from build123d import *

# Parameters (mm, degrees)
F1_DEPTH = 1.5
F3_DEPTH = 6.5
F4_R     = 0.1
F5_R     = 1
F6_R     = 1


# Not quite as in the source:
# - a feature of the source that left no trace in its solid (it failed there, or was rolled back) is left out


with BuildPart() as f1:
    # F0 (on Top) → F1 (new body)
    with BuildSketch(Plane.XY):
        with BuildLine():
            Line((13.5, -3.5), (13.5, 3))
            Line((13.5, 3), (1.7699947357, 3))
            ThreePointArc((1.7699947357, 3), (1.00332674, 2.4581115268), (1.2583103115, 1.5545594745))
            ThreePointArc((1.2583103115, 1.5545594745), (0.6431264076, -1.8937762339), (-1.9447626006, 0.466795916))
            ThreePointArc((-1.9447626006, 0.466795916), (-2.4990001073, 1.3711303598), (-3.4033345511, 0.8168928531))
            ThreePointArc((-3.4033345511, 0.8168928531), (-2.748556438, -2.1668958229), (0, -3.5))
            Line((0, -3.5), (1.7699947357, -3.5))
            Line((1.7699947357, -3.5), (13.5, -3.5))
        make_face()
    extrude(amount=F1_DEPTH)

    # F2 (on face) → F3 (join, through all)
    with BuildSketch(Plane.XZ.offset(3.5)):
        Polygon((5, 0), (3.5, 0), (3.5, -19.5), (13.5, -19.5), (13.5, -18), (5, -18), align=None)
    extrude(amount=-F3_DEPTH)

    # F4
    f4_edges = [f1.edges().sort_by_distance(p)[0] for p in [
        (5, -0.25, 0),
        (5, -0.25, -18),
    ]]
    fillet(f4_edges, radius=F4_R)

    # F5
    f5_edges = [f1.edges().sort_by_distance(p)[0] for p in [
        (3.5, -0.25, 0),
        (3.5, -0.25, -19.5),
    ]]
    fillet(f5_edges, radius=F5_R)

    # F6
    f6_edges = [f1.edges().sort_by_distance(p)[0] for p in [
        (13.5, -3.5, -18.75),
        (13.5, 3, -18.75),
        (13.5, -3.5, 0.75),
        (13.5, 3, 0.75),
    ]]
    fillet(f6_edges, radius=F6_R)


solid = f1.part
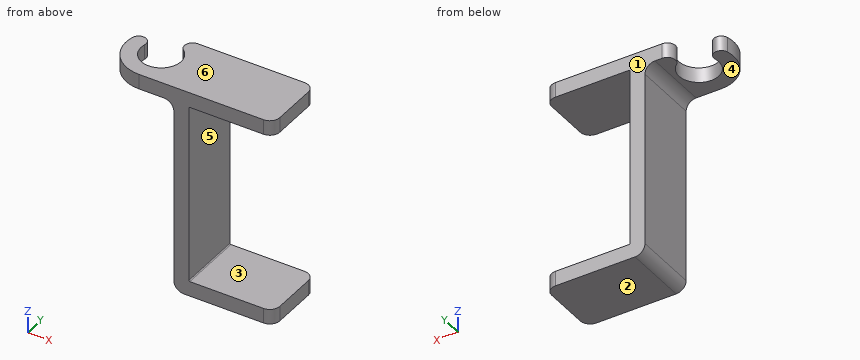
Model file for the job. Use its own axes, mm. Face numbers are marked on the shaded views. A direction names the side the tool comes from. Give positions to 0.01 mm unless a question says otherwise; leave off trailing zeros. Loops run counter-clockwise (first coordinate to the right, second up) from the corner with the lowest first, then second, coordinate; pieces in that order, holes last.
1) Flat gauge pins, fed straight in: pin 1 Ø2 at (y, z) = (-1, -5.5) entering from +X; pin 2 Ø2 at (x, y) = (-1.5, 1) entering from +Z; pin 3 Ø3 at (y, z) = (1, -14) entering from -X. Where does each tip first touch, or does it go through?
2) Pull direction Z, two halves, no side cores. Call the marked faces 1, 2 and 3: +Z half, -Z half, draft (parallel to the pull), parting line (faces both ways), or undercut.
3) Tool access for the marked faces 4, 5 and 6: list every direction of +Z, -Z, +X, -X, +Y, -Y with a clear straight run to the whole face (end or side of a thin tool).
4) Saw through at A-A (x = 6.5). Write the cut outline in (y, z).
5) Saw through at D-D (z = -14.5). Write the cut outline in (x, y).
6) Wall check: line 1 (Z direction, x = 11.25, y = -2); line 2 (X direction, y = 0, z = 1.05); line 3 (X direction, y = -0.25, z = -18.5). Give the ranges that are in metal, low to high.
7) Saw through at C-C (y = -1.75). Write the cut outline in (x, z).
8) Saw through at B-B (y = 0). Write the cut outline in (x, z), plus the area to 3 significant figures.
Answer block:
1. pin 1: stops at x = 5
1. pin 2: stops at z = 1.5
1. pin 3: stops at x = 3.5
2. face 1: draft
2. face 2: -Z half
2. face 3: undercut
3. face 4: -Z, -X, +Y, -Y
3. face 5: +X, +Y, -Y
3. face 6: +Z, +X, -X, +Y, -Y
4. outline: (-3.5, -19.5) - (3, -19.5) - (3, -18) - (-3.5, -18) - close; (-3.5, 0) - (3, 0) - (3, 1.5) - (-3.5, 1.5) - close
5. outline: (3.5, -3.5) - (5, -3.5) - (5, 3) - (3.5, 3) - close
6. line 1: z = -19.5 to -18, 0 to 1.5
6. line 2: x = -3.5 to -2, 2 to 13.5
6. line 3: x = 3.5 to 13.5
7. outline: (-3.03, 0) - (-0.97, 0) - (-0.97, 1.5) - (-3.03, 1.5) - close; (0.97, 0) - (2.5, 0) arc R1 cw to (3.5, -1) - (3.5, -18.5) arc R1 ccw to (4.5, -19.5) - (13.5, -19.5) - (13.5, -18) - (5.1, -18) arc R0.1 cw to (5, -17.9) - (5, -0.1) arc R0.1 cw to (5.1, 0) - (13.5, 0) - (13.5, 1.5) - (0.97, 1.5) - close
8. outline: (-3.5, 0) - (-2, 0) - (-2, 1.5) - (-3.5, 1.5) - close; (2, 0) - (2.5, 0) arc R1 cw to (3.5, -1) - (3.5, -18.5) arc R1 ccw to (4.5, -19.5) - (13.5, -19.5) - (13.5, -18) - (5.1, -18) arc R0.1 cw to (5, -17.9) - (5, -0.1) arc R0.1 cw to (5.1, 0) - (13.5, 0) - (13.5, 1.5) - (2, 1.5) - close
8. area: 61.5 mm2
